Geometry: final body of the model. Coordinates: model frame, mm. A direction names the side the tool comes from. Coordinates: 2 decimals unless noted, no trailing zeros. Order: outer loops, then holes, each group sorted by start corner. A loop starts at its lowest first (then second) coordinate and runs counter-clockwise, first axis right, second up. Notation, with made-up numbers: (-2.5, 88.25) - (39.5, 88.25) arc R5 ccw to (39.5, 97.25) - close; hole circle Ø1 at (54.25, -15). An arc over 180 degrees is marked (long way). Use a Markdown table: item, result. Add a question column.
```python
from build123d import *

# Parameters (mm, degrees)
SKETCH1_R               = 35
SKETCH1_R_2             = 2.2
SKETCH1_R_3             = 10
BOSS_EXTRUDE1_DEPTH     = 5
ECHELLE2_SCALE          = 2
ESQUISSE3_R             = 5
ENL_V_MAT_EXTRU_1_DEPTH = 10
ECHELLE3_SCALE          = 0.25


with BuildPart() as part:
    # Sketch1 → Boss-Extrude1 (new body)
    with BuildSketch(Plane(origin=(0, 0, 0), x_dir=(1, 0, 0), z_dir=(0, 1, 0))):
        with Locations(Location((0, 0, 0), (0, 0, 270))):
            Circle(SKETCH1_R)
        with Locations(Location((0, 25, 0), (0, 0, 270))):
            Circle(SKETCH1_R_2, mode=Mode.SUBTRACT)
        with Locations(Location((25, 0, 0), (0, 0, 270))):
            Circle(SKETCH1_R_2, mode=Mode.SUBTRACT)
        with Locations(Location((0, -25, 0), (0, 0, 270))):
            Circle(SKETCH1_R_2, mode=Mode.SUBTRACT)
        with Locations(Location((-25, 0, 0), (0, 0, 270))):
            Circle(SKETCH1_R_2, mode=Mode.SUBTRACT)
        with Locations(Location((0, 0, 0), (0, 0, 270))):
            Circle(SKETCH1_R_3, mode=Mode.SUBTRACT)
    extrude(amount=BOSS_EXTRUDE1_DEPTH)


with BuildPart() as part_1:
    # Echelle2: scaled about (0, 2.5, 0)
    add(part.part.scale(ECHELLE2_SCALE).moved(Location((0, -2.5, 0))))

    # Esquisse3 → Enlèv. mat.-Extru.1 (cut)
    with BuildSketch(Plane.XZ.offset(2.5)):
        with Locations((16.717937413, 1.193862082)):
            Circle(ESQUISSE3_R)
        with Locations((-7.898828439, 15.335211041)):
            Circle(ESQUISSE3_R)
    extrude(amount=-ENL_V_MAT_EXTRU_1_DEPTH, mode=Mode.SUBTRACT)


with BuildPart() as part_2:
    # Echelle3: scaled about (-0.005350728, 2.5, -0.020561043)
    add(part_1.part.scale(ECHELLE3_SCALE).moved(Location((-0.004013046, 1.875, -0.015420782))))


solid = part_2.part
```
1) Pin query (flat end, axial travel): pin 1 (2 mm diameter, centred on x = 0, z = 12.48, fed in from -Y); pin 2 (3.5 mm diameter, centred on x = 0, z = -12.52, fed in from -Y); pin 3 (1.5 mm diameter, centred on y = 1.5, z = -4, fed in from +X); pin 4 (1 mm diameter, centred on y = 2, z = -14, fed in from -X). Return the tip coordinate at first contact, or that it passes through.
2) Section D-D (z = 5.5). Return loops of the section in (x, y).
3) Draft query along X for faces 1 (the face through (2.435, 2.482, 4.349)), 2 (the face through (5.423, 2.482, 0.355)), 3 (the face through (-4, 3.75, 4)), 4 (the face through (-17.088, 2.482, -3.809)). Return one class per face: pulls with the +X half, pulls with the -X half, needs draft (parallel to the pull), parting line crosses it, or undercut.
4) Section B-B (z = 12). Return loops of the section in (x, y), then the cut area to 3 significant figures.
5) Set-up query: faces 5 (the face through (-2.53, 2.48, 4.94)), 6 (the face through (-4, 1.25, 4)). Return all of +Z, -Z, +X, -X, +Y, -Y with unobstructed straight access to the full face (end or side cutting, diameter ignored); none if empty.
6) Section C-C (y = 2.8). Return loops of the section in (x, z), then the cut area to 3 significant figures.
7) Section A-A (x = 3). Return loops of the section in (y, z).
8) Ray query, line 1 along X through (y, z) = (3.6, 0); line 2 along Z through (x, y) = (-4.5, 2.8); line 3 along Z through (x, y) = (-12, 3.45). Return the intervals inside material, ascending.
Values follow:
| question | item | result |
|---|---|---|
| 1 | pin 1 | passes through |
| 1 | pin 2 | stops at y = 1.25 |
| 1 | pin 3 | stops at x = 17.19 |
| 1 | pin 4 | stops at x = -11.16 |
| 2 | outline | (-16.61, 1.25) - (16.6, 1.25) - (16.6, 3.75) - (-16.61, 3.75) - close |
| 3 | face 1 | undercut |
| 3 | face 2 | undercut |
| 3 | face 3 | needs draft |
| 3 | face 4 | parting line crosses it |
| 4 | outline | (-12.73, 1.25) - (-0.99, 1.25) - (-0.99, 3.75) - (-12.73, 3.75) - close; (0.98, 1.25) - (12.72, 1.25) - (12.72, 3.75) - (0.98, 3.75) - close |
| 4 | area | 58.7 mm² |
| 5 | face 5 | +Y, -Y |
| 5 | face 6 | +Z, -Z, +X, -X, -Y |
| 6 | outline | circle Ø35 at (0, -0.02); hole circle Ø2.2 at (-12.5, -0.02); hole (-3.23, 3.81) arc R5 ccw (long way) to (4.95, -0.7) arc R1.25 ccw to (4.8, 1.36) arc R5 ccw to (-1.24, 4.83) arc R1.25 ccw to start; hole circle Ø2.2 at (0, -12.52); hole circle Ø2.2 at (0, 12.48); hole circle Ø2.2 at (12.5, -0.02) |
| 6 | area | 867 mm² |
| 7 | outline | (1.25, -17.26) - (3.75, -17.26) - (3.75, -4.01) - (1.25, -4.01) - close; (1.25, 3.98) - (3.75, 3.98) - (3.75, 17.22) - (1.25, 17.22) - close |
| 8 | line 1 | x = -17.5 to -13.6, -11.4 to -5, 5.39 to 11.4, 13.6 to 17.5 |
| 8 | line 2 | z = -16.93 to -2.2, 2.17 to 16.9 |
| 8 | line 3 | z = -12.76 to -0.99, 0.96 to 12.73 |
